from build123d import *

# Parameters (mm, degrees)
SKETCH_1_R          = 71
EXTRUDE_1_DEPTH     = 20
SKETCH_2_R          = 50.75
EXTRUDE_2_DEPTH     = 24.5
SKETCH_4_R          = 31
CUT_EXTRUDE_1_DEPTH = 35
CHAMFER_1_SIZE      = 0.5
SKETCH_5_R          = 27
CUT_EXTRUDE_2_DEPTH = 8
SKETCH_6_R          = 31.5
CUT_EXTRUDE_3_DEPTH = 2
CUT_EXTRUDE_4_REACH = 105.355
SKETCH_7_R          = 4.5
SKETCH_8_R          = 4
CUT_EXTRUDE_5_DEPTH = 10
SKETCH_9_R          = 4.5
CUT_EXTRUDE_6_DEPTH = 12


with BuildPart() as part:
    # 草图1 → 凸台-拉伸1 (new body)
    with BuildSketch(Plane.XY):
        Circle(SKETCH_1_R)
    extrude(amount=EXTRUDE_1_DEPTH)

    # 草图2 → 凸台-拉伸2 (add)
    with BuildSketch(Plane.XY.offset(20)):
        Circle(SKETCH_2_R)
    extrude(amount=EXTRUDE_2_DEPTH)

    # 草图4 → 切除-拉伸1 (cut)
    with BuildSketch(Plane.XY.offset(44.5)):
        Circle(SKETCH_4_R)
    extrude(amount=-CUT_EXTRUDE_1_DEPTH, mode=Mode.SUBTRACT)

    # 倒角1
    chamfer_1_edges = [part.edges().sort_by_distance(p)[0] for p in [
        (-31, 0, 44.5),
        (-50.75, 0, 44.5),
    ]]
    chamfer(chamfer_1_edges, length=CHAMFER_1_SIZE)

    # 草图5 → 切除-拉伸2 (cut)
    with BuildSketch(Plane(origin=(0, 0, 0), x_dir=(-1, 0, 0), z_dir=(0, 0, -1))):
        Circle(SKETCH_5_R)
    extrude(amount=-CUT_EXTRUDE_2_DEPTH, mode=Mode.SUBTRACT)

    # 草图6 → 切除-拉伸3 (cut)
    with BuildSketch(Plane.XY.offset(9.5)):
        Circle(SKETCH_6_R)
    extrude(amount=-CUT_EXTRUDE_3_DEPTH, mode=Mode.SUBTRACT)

    # 草图7 → 切除-拉伸4 (cut, up to next)
    with BuildSketch(Plane.XY.offset(20), mode=Mode.PRIVATE) as cut_extrude_4_sk1:
        with Locations((-61, 0)):
            Circle(SKETCH_7_R)
    cut_extrude_4_tool1 = extrude(cut_extrude_4_sk1.sketch, amount=-CUT_EXTRUDE_4_REACH, mode=Mode.PRIVATE) & part.part
    # 草图7 → 切除-拉伸4 (cut, up to next)
    with BuildSketch(Plane.XY.offset(20), mode=Mode.PRIVATE) as cut_extrude_4_sk2:
        with Locations((-30.5, 52.827549631)):
            Circle(SKETCH_7_R)
    cut_extrude_4_tool2 = extrude(cut_extrude_4_sk2.sketch, amount=-CUT_EXTRUDE_4_REACH, mode=Mode.PRIVATE) & part.part
    # 草图7 → 切除-拉伸4 (cut, up to next)
    with BuildSketch(Plane.XY.offset(20), mode=Mode.PRIVATE) as cut_extrude_4_sk3:
        with Locations((30.5, 52.827549631)):
            Circle(SKETCH_7_R)
    cut_extrude_4_tool3 = extrude(cut_extrude_4_sk3.sketch, amount=-CUT_EXTRUDE_4_REACH, mode=Mode.PRIVATE) & part.part
    # 草图7 → 切除-拉伸4 (cut, up to next)
    with BuildSketch(Plane.XY.offset(20), mode=Mode.PRIVATE) as cut_extrude_4_sk4:
        with Locations((61, 0)):
            Circle(SKETCH_7_R)
    cut_extrude_4_tool4 = extrude(cut_extrude_4_sk4.sketch, amount=-CUT_EXTRUDE_4_REACH, mode=Mode.PRIVATE) & part.part
    # 草图7 → 切除-拉伸4 (cut, up to next)
    with BuildSketch(Plane.XY.offset(20), mode=Mode.PRIVATE) as cut_extrude_4_sk5:
        with Locations((30.5, -52.827549631)):
            Circle(SKETCH_7_R)
    cut_extrude_4_tool5 = extrude(cut_extrude_4_sk5.sketch, amount=-CUT_EXTRUDE_4_REACH, mode=Mode.PRIVATE) & part.part
    # 草图7 → 切除-拉伸4 (cut, up to next)
    with BuildSketch(Plane.XY.offset(20), mode=Mode.PRIVATE) as cut_extrude_4_sk6:
        with Locations((-30.5, -52.827549631)):
            Circle(SKETCH_7_R)
    cut_extrude_4_tool6 = extrude(cut_extrude_4_sk6.sketch, amount=-CUT_EXTRUDE_4_REACH, mode=Mode.PRIVATE) & part.part
    add(cut_extrude_4_tool1.solids().sort_by_distance((-61, 0, 20))[0], mode=Mode.SUBTRACT)
    add(cut_extrude_4_tool2.solids().sort_by_distance((-30.5, 52.82755, 20))[0], mode=Mode.SUBTRACT)
    add(cut_extrude_4_tool3.solids().sort_by_distance((30.5, 52.82755, 20))[0], mode=Mode.SUBTRACT)
    add(cut_extrude_4_tool4.solids().sort_by_distance((61, 0, 20))[0], mode=Mode.SUBTRACT)
    add(cut_extrude_4_tool5.solids().sort_by_distance((30.5, -52.82755, 20))[0], mode=Mode.SUBTRACT)
    add(cut_extrude_4_tool6.solids().sort_by_distance((-30.5, -52.82755, 20))[0], mode=Mode.SUBTRACT)

    # 草图8 → 切除-拉伸5 (cut)
    with BuildSketch(Plane(origin=(0, 0, 0), x_dir=(-1, 0, 0), z_dir=(0, 0, -1))):
        with Locations((-41, 0)):
            Circle(SKETCH_8_R)
    extrude(amount=-CUT_EXTRUDE_5_DEPTH, mode=Mode.SUBTRACT)

    # 草图9 → 切除-拉伸6 (cut)
    with BuildSketch(Plane.XY.offset(44.5)):
        with Locations((41, 0)):
            Circle(SKETCH_9_R)
        with Locations((20.5, -35.507041555)):
            Circle(SKETCH_9_R)
        with Locations((-20.5, -35.507041555)):
            Circle(SKETCH_9_R)
        with Locations((-41, 0)):
            Circle(SKETCH_9_R)
        with Locations((-20.5, 35.507041555)):
            Circle(SKETCH_9_R)
        with Locations((20.5, 35.507041555)):
            Circle(SKETCH_9_R)
    extrude(amount=-CUT_EXTRUDE_6_DEPTH, mode=Mode.SUBTRACT)


solid = part.part
The listing builds one solid part. Answer for the finished solid, in the listing's coordinates (mm). A direction names the side the tool comes from. Coordinates: 2 decimals unless noted, no trailing zeros. Write each loop counter-clockwise with the first axis right and the second up, starting at its lowest first coordinate (ties: lowest second). Pieces come first, ordered by that corner, then holes. Notation, with made-up numbers: (71.25, -29.75) - (111.25, -29.75) arc R26 ccw to (111.25, 6.25) - close; hole circle Ø10 at (52, 87). An arc over 180 degrees is marked (long way). Answer as CSV lines item,"result".
1. Find section B-B (z = 17). Give the vertices of the cut face in (x, y), plus the area to 3 significant figures.
Computed values:
outline,"circle Ø142 at (0, 0); hole circle Ø9 at (-61, 0); hole circle Ø9 at (-30.5, -52.83); hole circle Ø9 at (-30.5, 52.83); hole circle Ø62 at (0, 0); hole circle Ø9 at (30.5, -52.83); hole circle Ø9 at (30.5, 52.83); hole circle Ø9 at (61, 0)"
area,"12,400 mm²"
2. Given P1, Ø7, axis at x = 20.5, y = 35.51, coming from the +Z side; P2, Ø2, axis at x = 17.5, z = 8.5, coming from the +Y side; P3, Ø3, axis at y = -41.5, z = 16, coming from the -X side, each flat-ended and moving along its own axis, determine where each tip first touches the part or whether it passes through.
Computed values:
P1,"stops at z = 32.5"
P2,"stops at y = 69.06"
P3,"stops at x = -58.66"
3. Determine the mould class of faces 1 (the flat face through (20.9, -23.2, 9.5)), 2 (the cylindrical face through (16.929, -38.245, 38.584)), 3 (the flat face through (41, 0, 32.5)), 4 (the flat face through (41, 0, 10)) for opening direction Z: +Z half, -Z half, draft (parallel to the pull), parting line (faces both ways), or undercut.
Computed values:
face 1,"undercut"
face 2,"draft"
face 3,"+Z half"
face 4,"-Z half"
4. Find section A-A (x = 0). Give the vertices of the cut face in (y, z).
Computed values:
outline,"(-71, 0) - (-27, 0) - (-27, 7.5) - (-31.5, 7.5) - (-31.5, 9.5) - (-31, 9.5) - (-31, 44) - (-31.5, 44.5) - (-50.25, 44.5) - (-50.75, 44) - (-50.75, 20) - (-71, 20) - close; (27, 0) - (71, 0) - (71, 20) - (50.75, 20) - (50.75, 44) - (50.25, 44.5) - (31.5, 44.5) - (31, 44) - (31, 9.5) - (31.5, 9.5) - (31.5, 7.5) - (27, 7.5) - close"
5. Straight lines are drawn through the part: line 1 (Z direction, x = -55.5, y = -26); line 2 (Y direction, x = 65, z = 2); line 3 (Y direction, x = -64, z = 6.5). For each, find the intervals that lie inside material, in ascending order. Write a range as [from, to].
Computed values:
line 1,"z = [0, 20]"
line 2,"y = [-28.57, -2.06], [2.06, 28.57]"
line 3,"y = [-30.74, -3.35], [3.35, 30.74]"
6. A tool of negligible diameter and unlimited length cuts with its end or side. For faces 5 (the flat face through (-21, -35, 32.5)), 6 (the cylindrical face through (-4.101, 31.232, 8.514)), 7 (the cylindrical face through (65.16, -1.72, 10.14)), 8 (the cylindrical face through (44.2, -2.4, 4.9)), from which of +Z, -Z, +X, -X, +Y, -Y can it reach the whole face along a straight path? Write none if from no direction.
Computed values:
face 5,"+Z"
face 6,"none"
face 7,"+Z, -Z"
face 8,"-Z"
7. Find section C-C (y = 0). Give the number of separate pieces and of enclosed holes in the cut face, plus the area to 3 significant figures.
Computed values:
separate pieces,"4"
enclosed holes,"0"
area,"1,970 mm²"
